```python
from build123d import *

# Parameters (mm, degrees)
F1_DEPTH = 400


with BuildPart() as f1:
    # F0 (on Front) → F1 (new body)
    with BuildSketch(Plane.XZ):
        with BuildLine():
            add(Edge.make_bspline(
                [(-349.9918261405, 164.7005370527), (-228.7541310859, 152.8680934101), (-148.4648335347, 151.7757154689), (0, 148.7712413073)],
                knots=[17.2755734709, 17.2755734709, 17.2755734709, 17.2755734709, 368.6136798781, 368.6136798781, 368.6136798781, 368.6136798781], degree=3))
            add(Edge.make_bspline(
                [(-349.9918261405, 164.7005370527), (-379.7747257767, 166.5833651071), (-400.0212253579, 152.0293008743), (-412.6107976831, 127.4847845064)],
                knots=[0, 0, 0, 0, 86.6035481416, 86.6035481416, 86.6035481416, 86.6035481416], degree=3))
            add(Edge.make_bspline(
                [(-412.6107976774, 127.4847845008), (-390.2805647898, 125.7630890537), (-367.6040024639, 124.021633923), (-344.5166107631, 122.3204635533)],
                knots=[55.3884070152, 55.3884070152, 55.3884070152, 55.3884070152, 129.1746995747, 129.1746995747, 129.1746995747, 129.1746995747], degree=3))
            add(Edge.make_bspline(
                [(-332.2621001683, 121.4244425258), (-336.5916827882, 122.5915718518), (-340.6786149646, 122.8620951072), (-344.5166107631, 122.3204635533)],
                knots=[0, 0, 0, 0, 17.888080119, 17.888080119, 17.888080119, 17.888080119], degree=3))
            add(Edge.make_bspline(
                [(-332.2621001683, 121.4244425258), (-231.2540764526, 114.0987320503), (-122.2665528935, 107.7345344123), (0, 107.2653010488)],
                knots=[142.1884395148, 142.1884395148, 142.1884395148, 142.1884395148, 462.9643141605, 462.9643141605, 462.9643141605, 462.9643141605], degree=3))
            add(Edge.make_bspline(
                [(332.2621001683, 121.4244425258), (231.2540764526, 114.0987320503), (122.2665528935, 107.7345344123), (0, 107.2653010488)],
                knots=[142.1884395148, 142.1884395148, 142.1884395148, 142.1884395148, 462.9643141605, 462.9643141605, 462.9643141605, 462.9643141605], degree=3))
            add(Edge.make_bspline(
                [(332.2621001683, 121.4244425258), (336.5916827882, 122.5915718518), (340.6786149646, 122.8620951072), (344.5166107631, 122.3204635533)],
                knots=[0, 0, 0, 0, 17.888080119, 17.888080119, 17.888080119, 17.888080119], degree=3))
            add(Edge.make_bspline(
                [(412.6107976774, 127.4847845008), (390.2805647898, 125.7630890537), (367.6040024639, 124.021633923), (344.5166107631, 122.3204635533)],
                knots=[55.3884070152, 55.3884070152, 55.3884070152, 55.3884070152, 129.1746995747, 129.1746995747, 129.1746995747, 129.1746995747], degree=3))
            add(Edge.make_bspline(
                [(349.9918261405, 164.7005370527), (379.7747257767, 166.5833651071), (400.0212253579, 152.0293008743), (412.6107976831, 127.4847845064)],
                knots=[0, 0, 0, 0, 86.6035481416, 86.6035481416, 86.6035481416, 86.6035481416], degree=3))
            add(Edge.make_bspline(
                [(349.9918261405, 164.7005370527), (228.7541310859, 152.8680934101), (148.4648335347, 151.7757154689), (0, 148.7712413073)],
                knots=[17.2755734709, 17.2755734709, 17.2755734709, 17.2755734709, 368.6136798781, 368.6136798781, 368.6136798781, 368.6136798781], degree=3))
        make_face()
        with BuildLine():
            add(Edge.make_bspline(
                [(-412.6107976774, 127.4847845008), (-390.2805647898, 125.7630890537), (-367.6040024639, 124.021633923), (-344.5166107631, 122.3204635533)],
                knots=[55.3884070152, 55.3884070152, 55.3884070152, 55.3884070152, 129.1746995747, 129.1746995747, 129.1746995747, 129.1746995747], degree=3))
            add(Edge.make_bspline(
                [(-412.6107976831, 127.4847845064), (-455.2641858876, 44.3281245427), (-410.0275390456, -153.5039344324), (-349.9918261405, -215.3152623841)],
                knots=[86.6035481416, 86.6035481416, 86.6035481416, 86.6035481416, 380.0157994368, 380.0157994368, 380.0157994368, 380.0157994368], degree=3))
            add(Edge.make_bspline(
                [(-349.9918261405, -215.3152623841), (-287.5397462749, -281.8407177446), (-155.7662200923, -118.8372276745), (0, -119.0087459604)],
                knots=[0, 0, 0, 0, 363.0003078109, 363.0003078109, 363.0003078109, 363.0003078109], degree=3))
            add(Edge.make_bspline(
                [(349.9918261405, -215.3152623841), (287.5397462749, -281.8407177446), (155.7662200923, -118.8372276745), (0, -119.0087459604)],
                knots=[0, 0, 0, 0, 363.0003078109, 363.0003078109, 363.0003078109, 363.0003078109], degree=3))
            add(Edge.make_bspline(
                [(412.6107976831, 127.4847845064), (455.2641858876, 44.3281245427), (410.0275390456, -153.5039344324), (349.9918261405, -215.3152623841)],
                knots=[86.6035481416, 86.6035481416, 86.6035481416, 86.6035481416, 380.0157994368, 380.0157994368, 380.0157994368, 380.0157994368], degree=3))
            add(Edge.make_bspline(
                [(412.6107976774, 127.4847845008), (390.2805647898, 125.7630890537), (367.6040024639, 124.021633923), (344.5166107631, 122.3204635533)],
                knots=[55.3884070152, 55.3884070152, 55.3884070152, 55.3884070152, 129.1746995747, 129.1746995747, 129.1746995747, 129.1746995747], degree=3))
            add(Edge.make_bspline(
                [(344.5166107631, 122.3204635533), (404.847274862, 113.8063866609), (403.6665423185, -95.3885912359), (316.5586292744, -177.2394478321)],
                knots=[17.888080119, 17.888080119, 17.888080119, 17.888080119, 299.0764424053, 299.0764424053, 299.0764424053, 299.0764424053], degree=3))
            add(Edge.make_bspline(
                [(316.5586292744, -177.2394478321), (289.4581258297, -209.2567682266), (174.6161052003, -83.5422830285), (0, -86.466948735)],
                knots=[0, 0, 0, 0, 329.3159764731, 329.3159764731, 329.3159764731, 329.3159764731], degree=3))
            add(Edge.make_bspline(
                [(-316.5586292744, -177.2394478321), (-289.4581258297, -209.2567682266), (-174.6161052003, -83.5422830285), (0, -86.466948735)],
                knots=[0, 0, 0, 0, 329.3159764731, 329.3159764731, 329.3159764731, 329.3159764731], degree=3))
            add(Edge.make_bspline(
                [(-344.5166107631, 122.3204635533), (-404.847274862, 113.8063866609), (-403.6665423185, -95.3885912359), (-316.5586292744, -177.2394478321)],
                knots=[17.888080119, 17.888080119, 17.888080119, 17.888080119, 299.0764424053, 299.0764424053, 299.0764424053, 299.0764424053], degree=3))
        make_face()
    extrude(amount=F1_DEPTH)


solid = f1.part
```
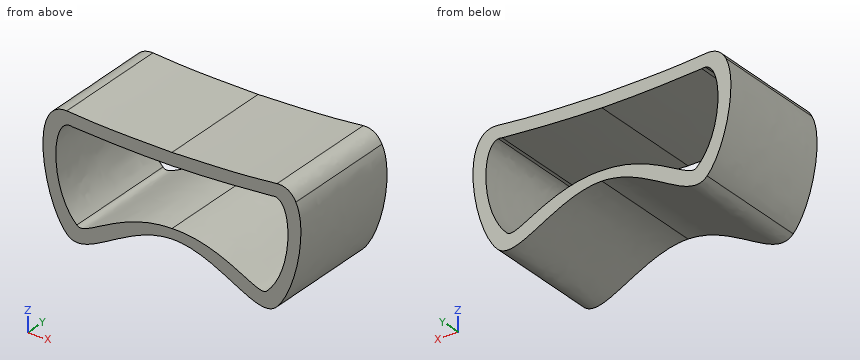
Verification items for the finished model (mm, model axes). Give positions to 0.01 mm unless a question says otherwise; leave off trailing zeros. Return JSON: item names as keys, results as strings. Group by question number.
1) Go/stop test with flat-tipped pins: pin 1 Ø1 at (x, y) = (50, -45) entering from -Z; pin 2 Ø2 at (y, z) = (-269, -32) entering from -X; pin 3 Ø3 at (y, z) = (-356.5, -183.5) entering from +X. Record where each tip stops, or that it passes through.
2) Scan lines: line 1 (X direction, y = -42, z = 52.5); line 2 (X direction, y = -127, z = -214); line 3 (X direction, y = -43, z = -167). Record each from-to range of solid material in increasing order.
3) Section check A-A on z = -136.5. Give the number of separate pieces and of enclosed holes in the cut face, and give its area (3 significant figures).
Answer block:
{
 "1": {"pin 1": "stops at z = -124.36", "pin 2": "stops at x = -423.56", "pin 3": "stops at x = 374.16"},
 "2": {"line 1": "x = -429.1 to -384.37, 384.37 to 429.1", "line 2": "x = -351.25 to -252.81, 252.81 to 351.25", "line 3": "x = -382.14 to -326.45, -260.68 to -162.83, 162.83 to 260.68, 326.45 to 382.14"},
 "3": {"separate pieces": "4", "enclosed holes": "0", "area": "124,000 mm^2"}
}
